Geometry: final body of the model. Coordinates: model frame, mm. Face numbers are marked on the shaded views. A direction names the side the tool comes from. Round coordinates to 2 decimals unless told otherwise and drop trailing zeros. Order: outer loops, then holes, each group sorted by start corner. A loop starts at its lowest first (then second) coordinate and runs counter-clockwise, first axis right, second up. Notation, with made-up numbers: (66, 55.5) - (114, 55.5) arc R35 cw to (114, 87.5) - close; hole circle Ø10 at (-12.75, 6.25). An arc over 180 degrees is marked (long way). Put each result on its own line as item: value. Start each with the question number.
(1) Section C-C (x = -62). Output: boundary loops of the cut face in (y, z).
(2) Material intervals for L1, parallel to X at y = 8.6, z = -3; L2, parallel to X at y = 6.65, z = 21; L3, parallel to X at y = 7.6, z = 12, sorted ascending. Write a range as [from, to].
(3) Section B-B (z = 37.5). Output: boundary loops of the cut face in (x, y).
(4) Section A-A (y = 9.55). Output: boundary loops of the cut face in (x, z) (1 decimal).
(5) Section D-D (x = -70). Output: boundary loops of the cut face in (y, z), and give its area (3 significant figures).
(6) Pin query (flat end, axial travel): P1, Ø1, axis at x = -55.5, y = 10, coming from the +Z side; P2, Ø1.8, axis at x = -61, y = 9.5, coming from the -Z side. Return the tip coordinate at first contact, or that it passes through.
(7) Pull-direction query (Z, two-part tool) for the marked faces 5, 6 and 7; classes: released by +Z, released by -Z, zero draft, split by the parting line, or undercut.
(8) Access query for the marked faces 1, 2, 3 and 4. Directions: +Z, -Z, +X, -X, +Y, -Y. A direction counts if a zero-diameter tool reaches every point of the face in a straight line with its end or side. Return the directions, or none.
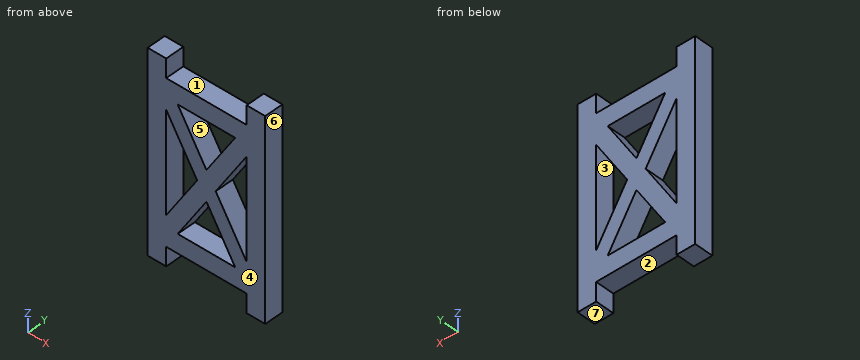
Autodesk Inventor part; units mm, degrees
ref_plane "YZ Plane" through (0, 0, 0) normal (1, 0, 0) x (0, 1, 0)
ref_plane "XZ Plane" through (0, 0, 0) normal (0, 1, 0) x (-1, 0, 0)
ref_plane "XY Plane" through (0, 0, 0) normal (0, 0, 1) x (1, 0, 0)
ref_plane "Work Plane2" through (-47, 12, 0) normal (0, -1, 0) x (0, 0, -1)
sketch "Sketch2" plane through (-47, 12, 0) normal (0, -1, 0) x (0, 0, -1)
  line L0 (0, 0) -> (0, 6)
  line L1 (0, 0) -> (6, 0)
  line L2 (6, 6) -> (6, 0)
  line L3 (0, 6) -> (6, 6)
  line L4 (0, -32) -> (0, -26)
  line L5 (0, -32) -> (6, -32)
  line L6 (6, -26) -> (6, -32)
  line L7 (0, -26) -> (6, -26)
  line L8 (-57.6, -32) -> (-57.6, -26)
  line L9 (-57.6, -32) -> (-51.6, -32)
  line L10 (-51.6, -26) -> (-51.6, -32)
  line L11 (-57.6, -26) -> (-51.6, -26)
  line L12 (-57.6, 0) -> (-57.6, 6)
  line L13 (-57.6, 0) -> (-51.6, 0)
  line L14 (-51.6, 6) -> (-51.6, 0)
  line L15 (-57.6, 6) -> (-51.6, 6)
  line L16 (-51.6, 6) -> (0, 6)
  line L17 (0, 0) -> (-51.6, 0)
  line L18 (-51.6, 0) -> (0, -32)
  line L19 (0, -26) -> (-51.6, 6)
  line L20 (-51.6, -32) -> (0, 0)
  line L21 (-51.6, -26) -> (0, 6)
  line L22 (0, -32) -> (-51.6, -32)
  line L23 (-51.6, -26) -> (0, -26)
  line L24 (-6, 0) -> (-6, -26)
  line L25 (0, 0) -> (0, -26)
  line L26 (-45.6, -26) -> (-45.6, 0)
  line L27 (-51.6, 0) -> (-51.6, -26)
  point P0 (0, 47)
  point P1 (-20.9625, -13)
  point P2 (-6, -3.7209)
  point P3 (-6, -22.2791)
  point P4 (-25.8, -10)
  point P5 (-41.925, 0)
  point P6 (-9.675, 0)
  point P7 (-25.8, -16)
  point P8 (-9.675, -26)
  point P9 (-41.925, -26)
  point P10 (-30.6375, -13)
  point P11 (-45.6, -22.2791)
  point P12 (-45.6, -3.7209)
extrude "Extrusion1" add sketch "Sketch2" along normal blind 6 contours L17 L21 L0 | L0 L3 L2 L1 | L20 L24 L17 | L25 L19 L24 L20 | L21 L17 L19 L16 | L24 L20 L19 L21 L17 | L7 L6 L5 L4 | L23 L24 L19 | L4 L18 L23 | L19 L17 L14 | L14 L13 L12 L15 | L20 L18 L21 L19 | L19 L24 L23 L18 L20 | L22 L20 L23 L18 | L17 L26 L18 | L18 L26 L21 L27 | L19 L21 L18 L26 L17 | L20 L23 L26 L21 L18 | L9 L8 L11 L10 | L10 L23 L20 | L21 L26 L23
properties part number "CrossReinforcementUpper"
Checks:
1. outline: (6, 0) - (12, 0) - (12, 6) - (6, 6) - close; (6, 17.74) - (12, 17.74) - (12, 33.86) - (6, 33.86) - close; (6, 45.6) - (12, 45.6) - (12, 51.6) - (6, 51.6) - close
2. L1: x = [-79, -73], [-47, -41]
2. L2: x = [-79, -73], [-65.98, -54.02], [-47, -41]
2. L3: x = [-79, -73], [-71.56, -65.56], [-54.44, -48.44], [-47, -41]
3. outline: (-79, 6) - (-73, 6) - (-73, 12) - (-79, 12) - close; (-70.26, 6) - (-64.26, 6) - (-64.26, 12) - (-70.26, 12) - close; (-55.74, 6) - (-49.74, 6) - (-49.74, 12) - (-55.74, 12) - close; (-47, 6) - (-41, 6) - (-41, 12) - (-47, 12) - close
4. outline: (-79, -6) - (-73, -6) - (-73, 0) - (-47, 0) - (-47, -6) - (-41, -6) - (-41, 57.6) - (-47, 57.6) - (-47, 51.6) - (-73, 51.6) - (-73, 57.6) - (-79, 57.6) - close; hole (-73, 9.7) - (-63, 25.8) - (-73, 41.9) - close; hole (-69.3, 6) - (-50.7, 6) - (-60, 21) - close; hole (-69.3, 45.6) - (-60, 30.6) - (-50.7, 45.6) - close; hole (-57, 25.8) - (-47, 9.7) - (-47, 41.9) - close
5. outline: (6, 0) - (12, 0) - (12, 14.51) - (6, 14.51) - close; (6, 37.09) - (12, 37.09) - (12, 51.6) - (6, 51.6) - close
5. area: 174 mm²
6. P1: stops at z = 51.6
6. P2: stops at z = 0
7. face 5: undercut
7. face 6: zero draft
7. face 7: released by -Z
8. face 1: +Z, +Y, -Y
8. face 2: -Z, +Y, -Y
8. face 3: +Y, -Y
8. face 4: +Z, -Z, +X, -X, -Y
